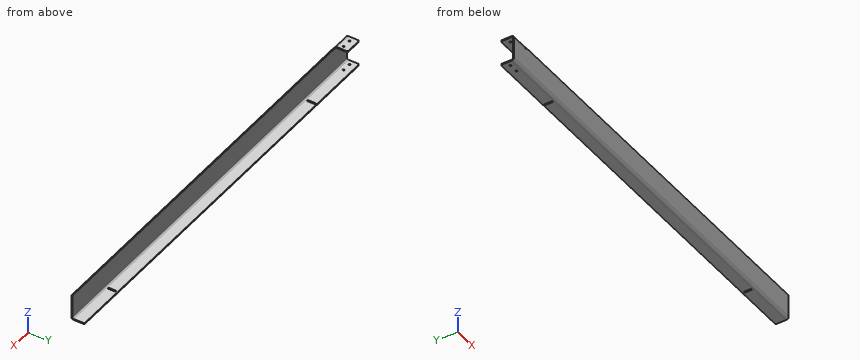
```python
from build123d import *

# Parameters (mm, degrees)
SKETCH1_W                     = 1209.675
SKETCH1_H                     = 72.39
BASE_FLANGE1_DEPTH            = 3.175
EDGE_FLANGE1_STRIP_W          = 20.32
EDGE_FLANGE1_STRIP_H          = 3.175
EDGE_FLANGE1_STRIP_CUT_DEPTH  = 1209.675
EDGE_FLANGE1_DEPTH            = 1209.675
SKETCH10_W                    = 4.191
SKETCH10_H                    = 22.225
CUT_EXTRUDE2_DEPTH            = 611.344430225
EDGE_FLANGE2_STRIP_W          = 20.32
EDGE_FLANGE2_STRIP_H          = 3.175
EDGE_FLANGE2_STRIP_CUT_DEPTH  = 50.8
EDGE_FLANGE2_RELIEF_W         = 21.9075
EDGE_FLANGE2_RELIEF_H         = 1.5875
EDGE_FLANGE2_RELIEF_CUT_DEPTH = 3.175
EDGE_FLANGE2_DEPTH            = 50.8
F_10_0_1935_DIAMETER_HOLE1_D  = 4.9149
FILLET1_R                     = 3.175
LPATTERN1_COUNT               = 2
LPATTERN1_PITCH               = 876.173


# Sheet-metal steps are written as plain solids
with BuildPart() as part:
    # Sketch1 → Base-Flange1 (new body)
    with BuildSketch(Plane(origin=(0, 0, 0), x_dir=(1, 0, 0), z_dir=(0, 1, 0))):
        with Locations((0, -36.195)):
            Rectangle(SKETCH1_W, SKETCH1_H)
    extrude(amount=BASE_FLANGE1_DEPTH)

    # Edge-Flange1 strip (across the edge) → Edge-Flange1 strip cut (cut)
    with BuildSketch(Plane(origin=(604.8375, 3.175, 0), x_dir=(0, 0, 1), z_dir=(-1, 0, 0))):
        with Locations((-3.175, -1.5875)):
            Rectangle(EDGE_FLANGE1_STRIP_W, EDGE_FLANGE1_STRIP_H)
    extrude(amount=EDGE_FLANGE1_STRIP_CUT_DEPTH, mode=Mode.SUBTRACT)

    # Edge-Flange1 section (across the edge) → Edge-Flange1 (add)
    with BuildSketch(Plane(origin=(604.8375, 3.175, 0), x_dir=(0, 0, 1), z_dir=(-1, 0, 0))):
        with BuildLine():
            Line((0, 3.81), (0, 34.925))
            Line((0, 34.925), (3.175, 34.925))
            Line((3.175, 34.925), (3.175, 3.81))
            ThreePointArc((3.175, 3.81), (4.290923164, 1.115923164), (6.985, 0))
            Line((6.985, 0), (6.985, -3.175))
            ThreePointArc((6.985, -3.175), (2.045859133, -1.129140867), (0, 3.81))
        make_face()
    extrude(amount=EDGE_FLANGE1_DEPTH)

    # Sketch10 → Cut-Extrude2 (cut, through all)
    with BuildSketch(Plane(origin=(0, 0, 0), x_dir=(-1, 0, 0), z_dir=(0, 0, -1))):
        with Locations((417.449, 22.225)):
            Rectangle(SKETCH10_W, SKETCH10_H)
    cut_extrude2 = extrude(amount=-CUT_EXTRUDE2_DEPTH, mode=Mode.SUBTRACT)

    # Edge-Flange2 strip (across the edge) → Edge-Flange2 strip cut (cut)
    with BuildSketch(Plane(origin=(-604.8375, 3.175, 72.39), x_dir=(0, 0, -1), z_dir=(1, 0, 0))):
        with Locations((-6.35, -1.5875)):
            Rectangle(EDGE_FLANGE2_STRIP_W, EDGE_FLANGE2_STRIP_H)
    extrude(amount=EDGE_FLANGE2_STRIP_CUT_DEPTH, mode=Mode.SUBTRACT)

    # Edge-Flange2 relief (on the sheet) → Edge-Flange2 relief cut (cut)
    with BuildSketch(Plane(origin=(-604.8375, 3.175, 68.58), x_dir=(0, 0, -1), z_dir=(0, 1, 0))):
        with Locations((-9.36625, -51.59375)):
            Rectangle(EDGE_FLANGE2_RELIEF_W, EDGE_FLANGE2_RELIEF_H)
    extrude(amount=-EDGE_FLANGE2_RELIEF_CUT_DEPTH, mode=Mode.SUBTRACT)

    # Edge-Flange2 section (across the edge) → Edge-Flange2 (add)
    with BuildSketch(Plane(origin=(-604.8375, 3.175, 72.39), x_dir=(0, 0, -1), z_dir=(1, 0, 0))):
        with BuildLine():
            Line((-3.175, 3.81), (-3.175, 34.925))
            Line((-3.175, 34.925), (0, 34.925))
            Line((0, 34.925), (0, 3.81))
            ThreePointArc((0, 3.81), (1.115923164, 1.115923164), (3.81, 0))
            Line((3.81, 0), (3.81, -3.175))
            ThreePointArc((3.81, -3.175), (-1.129140867, -1.129140867), (-3.175, 3.81))
        make_face()
    extrude(amount=EDGE_FLANGE2_DEPTH)

    # #10 (0.1935) Diameter Hole1 (through all)
    with Locations(Plane.XY.offset(75.565)):
        with Locations((-565.15, 19.05), (-590.55, 19.05)):
            Hole(F_10_0_1935_DIAMETER_HOLE1_D / 2)

    # Fillet1
    fillet1_edges = [part.edges().sort_by_distance(p)[0] for p in [
        (-604.8375, 38.1, 73.9775),
        (-554.0375, 38.1, 73.9775),
        (604.8375, 38.1, 1.5875),
        (-604.8375, 38.1, 1.5875),
        (604.8375, 1.5875, 72.39),
    ]]
    fillet(fillet1_edges, radius=FILLET1_R)

    # LPattern1: Cut-Extrude2 ×2
    with Locations(*[(i * LPATTERN1_PITCH, 0, 0) for i in range(1, LPATTERN1_COUNT)]):
        add(cut_extrude2, mode=Mode.SUBTRACT)


solid = part.part
```
Work out the finished part from the listing and answer in its coordinate system (mm). Give positions to 0.01 mm unless a question says otherwise; leave off trailing zeros. Order: outer loops, then holes, each group sorted by start corner. A loop starts at its lowest first (then second) coordinate and runs counter-clockwise, first axis right, second up. Notation, with made-up numbers: (39, 80.25) -> (54, 80.25) arc R22 ccw to (54, 107.25) -> close; hole circle Ø2 at (18, 47). An arc over 180 degrees is marked (long way). Answer as CSV lines item,"result". Start each with the question number.
(1) Each of these flat-tipped pins is pushed along its axis until it touches: pin 1 Ø4 at (x, y) = (-565.15, 19.05) entering from +Z; pin 2 Ø3.5 at (x, z) = (-417, 1) entering from -Y; pin 3 Ø2.5 at (x, y) = (161, 1.5) entering from +Z; pin 4 Ø1 at (x, z) = (122, 50.5) entering from +Y (3 decimals). Where does it stop, or does it pass through?
(2) Section A-A, the plane x = 9.5 is taken. Write down the section's boundary in (y, z) (3 decimals).
(3) Section B-B, the plane z = 22 is taken. Write down the section's boundary in (x, y) (1 decimal), plus the area to 3 significant figures.
(4) Consider line 1 along X through (y, z) = (19, 2); line 2 along Y through (x, z) = (-590.55, 74.3); line 3 along Z through (x, y) = (-139.5, 13) (3 decimals). Determine where each line is inside the solid, lowest interval first.
Entries:
1,pin 1,"through"
1,pin 2,"y = 1.43"
1,pin 3,"z = 72.39"
1,pin 4,"y = 3.175"
2,outline,"(0, 6.985) arc R6.985 ccw to (6.985, 0) -> (38.1, 0) -> (38.1, 3.175) -> (6.985, 3.175) arc R3.81 cw to (3.175, 6.985) -> (3.175, 72.39) -> (0, 72.39) -> close"
3,outline,"(-604.8, 0) -> (604.8, 0) -> (604.8, 3.2) -> (-604.8, 3.2) -> close"
3,area,"3,840 mm²"
4,line 1,"-604.84 to -593.01, -588.09 to -567.61, -562.69 to -419.54, -415.35 to 456.63, 460.82 to 604.84"
4,line 2,"2.98 to 16.59, 21.51 to 38.1"
4,line 3,"0 to 3.175"
